```python
from build123d import *

# Parameters (mm, degrees)
F1_DEPTH  = 38
F2_W      = 13
F2_H      = 4
F3_DEPTH  = 7.501
F4_W      = 16.0720253857
F4_H      = 15
F5_DEPTH  = 3
F6_W      = 16.0720253857
F6_H      = 15
F7_DEPTH  = 3
F9_DEPTH  = 16.05
F11_DEPTH = 16.05


with BuildPart() as f1:
    # F0 (on Front) → F1 (new body)
    with BuildSketch(Plane.XZ):
        Polygon((-13, 1.2), (-13, 0), (0, 0), (15.7895535086, -6.3), (15.7895535086, 1.2), align=None)
    extrude(amount=-F1_DEPTH)

    # F2 (on face) → F3 (cut, through all)
    with BuildSketch(Plane.XY.offset(1.2)):
        with Locations((-6.5, 33)):
            Rectangle(F2_W, F2_H)
        with Locations((-6.5, 27.5)):
            Rectangle(F2_W, F2_H)
        with Locations((-6.5, 22)):
            Rectangle(F2_W, F2_H)
        with Locations((-6.5, 16)):
            Rectangle(F2_W, F2_H)
        with Locations((-6.5, 10.5)):
            Rectangle(F2_W, F2_H)
        with Locations((-6.5, 5)):
            Rectangle(F2_W, F2_H)
        Polygon((15.7895535086, 3), (0, 0), (15.7895535086, 0), align=None)
        Polygon((15.7895535086, 38), (0, 38), (15.7895535086, 35), align=None)
    extrude(amount=-F3_DEPTH, mode=Mode.SUBTRACT)

    # F4 (on face) → F5 (join)
    with BuildSketch(Plane(origin=(6.9684065657, 36.676009446, 0), x_dir=(-0.9824246248, 0.186659735, 0), z_dir=(0.186659735, 0.9824246248, 0))):
        with Locations((-0.9429427615, -6.3)):
            Rectangle(F4_W, F4_H)
    extrude(amount=F5_DEPTH)

    # F6 (on face) → F7 (join)
    with BuildSketch(Plane(origin=(0, 0, 0), x_dir=(0.9824246248, 0.186659735, 0), z_dir=(0.186659735, -0.9824246248, 0))):
        Polygon((16.0720253857, -6.3), (0, 0), (0, -13.8), (16.0720253857, -13.8), align=None)
        with Locations((8.0360126929, -6.3)):
            Rectangle(F6_W, F6_H)
    extrude(amount=F7_DEPTH)

    # F8 (on face) → F9 (join)
    with BuildSketch(Plane(origin=(8.8211469429, -1.676009446, 0), x_dir=(0.186659735, 0.9824246248, 0), z_dir=(0.9824246248, -0.186659735, 0))):
        with BuildLine():
            Line((37.3321357405, -11.05), (37.3321357405, -9.05))
            ThreePointArc((37.3321357405, -9.05), (36.3321357405, -10.05), (37.3321357405, -11.05))
        make_face()
    extrude(amount=-F9_DEPTH)

    # F10 (on face) → F11 (join)
    with BuildSketch(Plane(origin=(15.7895535086, 3, 0), x_dir=(-0.186659735, 0.9824246248, 0), z_dir=(0.9824246248, 0.186659735, 0))):
        with BuildLine():
            Line((0, -9.05), (0, -11.05))
            ThreePointArc((0, -11.05), (1, -10.05), (0, -9.05))
        make_face()
    extrude(amount=-F11_DEPTH)


solid = f1.part
```
Read the model definition and answer for the solid it produces. Units are mm, in the model's axes. A direction names the side the tool comes from. Give positions to 0.01 mm unless a question says otherwise; leave off trailing zeros. Order: outer loops, then holes, each group sorted by start corner. A loop starts at its lowest first (then second) coordinate and runs counter-clockwise, first axis right, second up. Notation, with made-up numbers: (-28, 64) -> (-19, 64) arc R19 ccw to (-19, 82) -> close; hole circle Ø7 at (81.25, 52). An arc over 180 degrees is marked (long way). One line per item, written item: value. Start each with the question number.
(1) Flat-ended cylindrical pins translate along their axes: P1, Ø3.5, axis at x = -5.5, y = 36, coming from the -Z side; P2, Ø6, axis at x = 12, y = 20.5, coming from the -Z side; P3, Ø2, axis at y = 35, z = -7, coming from the +X side. Find the tip coordinate at first contact, or state that the pin passes through.
(2) The part is cut by section C-C (y = 6). Determine the outline of the cut face in (x, z), and give its area (3 significant figures).
(3) The part is cut by section B-B (z = -12.5). Determine the outline of the cut face in (x, y), and give its area (3 significant figures).
(4) Straight lines are drawn through the part: L1, parallel to Y at x = 6.5, z = -3.75 (3 decimals); L2, parallel to Y at x = 4, z = -8; L3, parallel to Y at x = 11.25, z = -1.25. For each, find the intervals that lie inside material, in ascending order.
(5) The part is cut by section D-D (z = -1.75). Determine the outline of the cut face in (x, y), and give its area (3 significant figures).
(6) A tool of negligible diameter and unlimited length cuts with its end or side. For faces 1 (the flat face through (-7, 13, 0)), 2 (the flat face through (-13, 13, 1)), 3 (the flat face through (6.03, 1.146, -8.337)), 4 (the flat face through (-7, 12.5, 1)), from which of +Z, -Z, +X, -X, +Y, -Y can it reach the whole face along a straight path? Write none if from no direction.
(7) The part is cut by section A-A (x = -5.5). Determine the outline of the cut face in (y, z).
Taken from the geometry:
1. P1: z = 0
1. P2: z = -5.98
1. P3: x = 15.98
2. outline: (0, 0) -> (15.79, -6.3) -> (15.79, 1.2) -> (0, 1.2) -> close
2. area: 68.7 mm^2
3. outline: (0, 0) -> (0.56, -2.95) -> (16.35, 0.05) -> (15.79, 3) -> close; (0, 38) -> (15.79, 35) -> (16.35, 37.95) -> (0.56, 40.95) -> close
3. area: 96.4 mm^2
4. L1: -1.819 to 1.235, 36.765 to 39.819
4. L2: -2.29 to 0.76, 37.24 to 40.29
4. L3: -0.92 to 38.92
5. outline: (0, 0) -> (0.56, -2.95) -> (16.35, 0.05) -> (15.79, 3) -> (15.79, 35) -> (16.35, 37.95) -> (0.56, 40.95) -> (0, 38) -> (4.39, 37.17) -> (4.39, 0.83) -> close
5. area: 486 mm^2
6. face 1: -Z, -X, +Y, -Y
6. face 2: +Z, -Z, -X, +Y, -Y
6. face 3: -X
6. face 4: +Z, -Z, -X
7. outline: (0, 0) -> (3, 0) -> (3, 1.2) -> (0, 1.2) -> close; (7, 0) -> (8.5, 0) -> (8.5, 1.2) -> (7, 1.2) -> close; (12.5, 0) -> (14, 0) -> (14, 1.2) -> (12.5, 1.2) -> close; (18, 0) -> (20, 0) -> (20, 1.2) -> (18, 1.2) -> close; (24, 0) -> (25.5, 0) -> (25.5, 1.2) -> (24, 1.2) -> close; (29.5, 0) -> (31, 0) -> (31, 1.2) -> (29.5, 1.2) -> close; (35, 0) -> (38, 0) -> (38, 1.2) -> (35, 1.2) -> close
